Work out the finished part from the listing and answer in its coordinate system (mm). Face numbers are marked on the shaded views. A direction names the side the tool comes from. Round coordinates to 2 decimals unless told otherwise and drop trailing zeros. Write each loop counter-clockwise with the first axis right and the second up, starting at its lowest first coordinate (ties: lowest second). Pieces come first, ordered by that corner, then holes. Notation, with made-up numbers: (52.25, 76) - (80.25, 76) arc R20 ccw to (80.25, 115) - close; hole circle Ø1 at (5.5, 9.25). An arc over 180 degrees is marked (long way). Answer as a JSON object with one key per item and string values.
```python
from build123d import *

# Parameters (mm, degrees)
F0_W      = 254
F0_H      = 203.2
F1_DEPTH  = 12.7
F2_R      = 4.445
F3_DEPTH  = 25.4
F4_W      = 50.8
F4_H      = 101.6
F5_DEPTH  = 6.35
F6_W      = 6.35
F6_H      = 101.6
F7_DEPTH  = 44.45
F8_R      = 4.445
F9_DEPTH  = 25.4
F10_R     = 6.35
F11_DEPTH = 25.4


with BuildPart() as f1:
    # F0 (on Top) → F1 (new body)
    with BuildSketch(Plane.XY):
        Rectangle(F0_W, F0_H)
    extrude(amount=F1_DEPTH)

    # F2 (on face) → F3 (cut)
    with BuildSketch(Plane.XY.offset(12.7)):
        with Locations((-53.975, 25.4)):
            Circle(F2_R)
        with Locations((-53.975, -25.4)):
            Circle(F2_R)
        with Locations((53.975, -25.4)):
            Circle(F2_R)
        with Locations((53.975, 25.4)):
            Circle(F2_R)
    extrude(amount=-F3_DEPTH, mode=Mode.SUBTRACT)

    # F4 (on face) → F5 (join)
    with BuildSketch(Plane.XY.offset(12.7)):
        with Locations((-50.8, 0)):
            Rectangle(F4_W, F4_H)
    extrude(amount=F5_DEPTH)

    # F6 (on face) → F7 (join)
    with BuildSketch(Plane.XY.offset(19.05)):
        with Locations((-28.575, 0)):
            Rectangle(F6_W, F6_H)
    extrude(amount=F7_DEPTH)

    # F8 (on face) → F9 (cut)
    with BuildSketch(Plane.XY.offset(19.05)):
        with Locations((-53.975, 25.4)):
            Circle(F8_R)
        with Locations((-53.975, -25.4)):
            Circle(F8_R)
    extrude(amount=-F9_DEPTH, mode=Mode.SUBTRACT)

    # F10 (on face) → F11 (cut)
    with BuildSketch(Plane(origin=(-31.75, 0, 0), x_dir=(0, -1, 0), z_dir=(-1, 0, 0))):
        with Locations((0, 44.45)):
            Circle(F10_R)
    extrude(amount=-F11_DEPTH, mode=Mode.SUBTRACT)

    # F12: F1 across plane


with BuildPart() as f1_1:
    add(f1.part)
    add(f1.part.mirror(Plane.YZ))


solid = f1_1.part
```
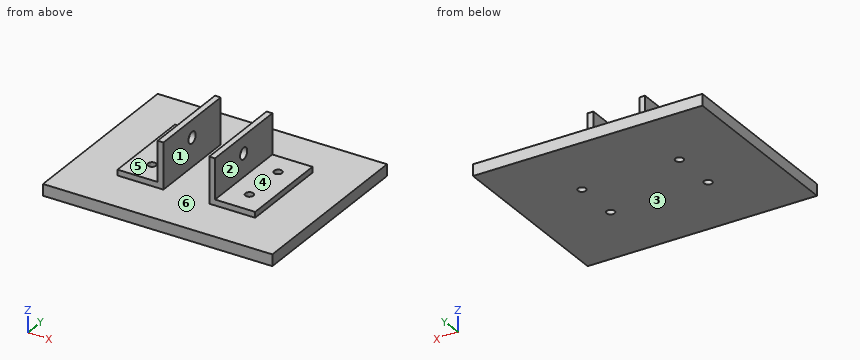
Item 1: A cutting plane is placed at D-D (x = 37.5). Write down the section's boundary in (y, z), and give its area (3 significant figures).
Results found:
{"outline": "(-101.6, 0) - (101.6, 0) - (101.6, 12.7) - (50.8, 12.7) - (50.8, 19.05) - (-50.8, 19.05) - (-50.8, 12.7) - (-101.6, 12.7) - close", "area": "3,230 mm²"}
Item 2: For the marked faces 4, 5 and 6, determine the directions among +Z, -Z, +X, -X, +Y, -Y from which every point of the face is accessible in a straight line to the end or side of a thin tool.
Results found:
{"face 4": "+Z, +X, +Y, -Y", "face 5": "+Z, -X, +Y, -Y", "face 6": "+Z"}
Item 3: Consider line 1 along X through (y, z) = (-25, 15); line 2 along X through (y, z) = (-5, 39.5); line 3 along Z through (x, y) = (-27, 0). Determine where each line is inside the solid, lowest interval first.
Results found:
{"line 1": "-76.2 to -58.4, -49.55 to -25.4, 25.4 to 49.55, 58.4 to 76.2", "line 2": "-31.75 to -25.4, 25.4 to 31.75", "line 3": "0 to 38.1, 50.8 to 63.5"}
Item 4: A cutting plane is placed at A-A (z = 44.45). Write down the section's boundary in (x, y).
Results found:
{"outline": "(-31.75, -50.8) - (-25.4, -50.8) - (-25.4, -6.35) - (-31.75, -6.35) - close; (-31.75, 6.35) - (-25.4, 6.35) - (-25.4, 50.8) - (-31.75, 50.8) - close; (25.4, -50.8) - (31.75, -50.8) - (31.75, -6.35) - (25.4, -6.35) - close; (25.4, 6.35) - (31.75, 6.35) - (31.75, 50.8) - (25.4, 50.8) - close"}
Item 5: Determine the mould class of the marked faces 1, 2 and 3 for opening direction X: pulls with the +X half, pulls with the -X half, needs draft (parallel to the pull), parting line crosses it, or undercut.
Results found:
{"face 1": "undercut", "face 2": "pulls with the +X half", "face 3": "needs draft"}
Item 6: A cutting plane is placed at C-C (z = 59). Write down the section's boundary in (x, y).
Results found:
{"outline": "(-31.75, -50.8) - (-25.4, -50.8) - (-25.4, 50.8) - (-31.75, 50.8) - close; (25.4, -50.8) - (31.75, -50.8) - (31.75, 50.8) - (25.4, 50.8) - close"}
Item 7: A cutting plane is placed at B-B (y = 0). Write down the section's boundary in (x, z), and give its area (3 significant figures).
Results found:
{"outline": "(-127, 0) - (127, 0) - (127, 12.7) - (76.2, 12.7) - (76.2, 19.05) - (31.75, 19.05) - (31.75, 38.1) - (25.4, 38.1) - (25.4, 12.7) - (-25.4, 12.7) - (-25.4, 38.1) - (-31.75, 38.1) - (-31.75, 19.05) - (-76.2, 19.05) - (-76.2, 12.7) - (-127, 12.7) - close; (-31.75, 50.8) - (-25.4, 50.8) - (-25.4, 63.5) - (-31.75, 63.5) - close; (25.4, 50.8) - (31.75, 50.8) - (31.75, 63.5) - (25.4, 63.5) - close", "area": "4,270 mm²"}
Item 8: Each of these flat-tipped pins is pushed along its axis until it touches: P1, Ø5, axis at y = 3.5, z = 15, coming from the +X side; P2, Ø14.5, axis at y = 0, z = 44.45, coming from the +X side; P3, Ø10, axis at x = 21, z = 39.5, coming from the +Y side; P4, Ø5, axis at y = -19.5, z = 22, coming from the -X side. Where does it stop, or does it pass through?
Results found:
{"P1": "x = 127", "P2": "x = 31.75", "P3": "y = 50.8", "P4": "x = -31.75"}
